```python
from build123d import *

# Parameters (mm, degrees)
SKETCH1_W                 = 15
SKETCH1_H                 = 15
BOSS_EXTRUDE1_DEPTH       = 3
SKETCH2_W                 = 8
SKETCH2_H                 = 3
CUT_EXTRUDE1_DEPTH        = 18.036725037
BOSS_EXTRUDE2_DEPTH       = 6
FILLET1_R                 = 2
CUT_EXTRUDE2_DEPTH        = 22.111371343
M3X0_5_TAPPED_HOLE1_D     = 2.5
M3X0_5_TAPPED_HOLE1_DEPTH = 7.5
M3X0_5_TAPPED_HOLE1_TIP   = 0.751075774
M3X0_5_TAPPED_HOLE2_D     = 2.5
M3X0_5_TAPPED_HOLE2_DEPTH = 7.5
M3X0_5_TAPPED_HOLE2_TIP   = 0.751075774


with BuildPart() as part:
    # Sketch1 → Boss-Extrude1 (new, symmetric)
    with BuildSketch(Plane.XY):
        Rectangle(SKETCH1_W, SKETCH1_H)
    extrude(amount=BOSS_EXTRUDE1_DEPTH, both=True)

    # Sketch2 → Cut-Extrude1 (cut, through all)
    with BuildSketch(Plane.XZ.offset(7.5)):
        Rectangle(SKETCH2_W, SKETCH2_H)
    extrude(amount=-CUT_EXTRUDE1_DEPTH, mode=Mode.SUBTRACT)

    # Sketch3 → Boss-Extrude2 (add)
    with BuildSketch(Plane.XY.offset(3)):
        with BuildLine():
            Line((7.5, -5.822370651), (7.5, 5.822370651))
            ThreePointArc((7.5, 5.822370651), (18.8, 0), (7.5, -5.822370651))
        make_face()
    extrude(amount=-BOSS_EXTRUDE2_DEPTH)

    # Fillet1
    # the kernel refuses this fillet: 2 mm, written as the material it adds along each edge
    with BuildSketch(Plane(origin=(7.5, -5.822370651, 3), x_dir=(0, -1, 0), z_dir=(0, 0, -1))) as fillet1_piece_1:
        with BuildLine():
            CenterArc((2.948715205, -1.544131065), FILLET1_R, 129.460264065, 67.086296359)
            ThreePointArc((1.031537969, -2.113719903), (0.603278499, -1.014153543), (0, 0))
            Line((0, 0), (1.677629349, 0))
        make_face()
    extrude(amount=6)
    with BuildSketch(Plane(origin=(7.5, 5.822370651, 3), x_dir=(0, 1, 0), z_dir=(0, 0, -1))) as fillet1_piece_2:
        with BuildLine():
            CenterArc((2.948715205, 1.544131065), FILLET1_R, 163.453439576, 67.086296359)
            ThreePointArc((1.031537969, 2.113719903), (0.603278499, 1.014153543), (0, 0))
            Line((0, 0), (1.677629349, 0))
        make_face()
    extrude(amount=6)
    # the kernel refuses this fillet: 2 mm, written as the material it takes off along each edge
    with BuildSketch(Plane(origin=(-7.5, -7.5, 8), x_dir=(1, 0, 0), z_dir=(0, 0, -1)), Plane(origin=(-7.5, 7.5, 8), x_dir=(0, -1, 0), z_dir=(0, 0, -1))) as fillet1_2_piece_1:
        with BuildLine():
            CenterArc((FILLET1_R, -FILLET1_R), FILLET1_R, 90, 90)
            Line((0, -FILLET1_R), (0, 0))
            Line((0, 0), (FILLET1_R, 0))
        make_face()
    extrude(amount=16, mode=Mode.SUBTRACT)

    # Sketch4 → Cut-Extrude2 (cut, through all)
    with BuildSketch(Plane(origin=(0, 0, -3), x_dir=(-1, 0, 0), z_dir=(0, 0, -1))):
        with BuildLine():
            Line((-18.8, 3), (-14.517490192, 3))
            ThreePointArc((-14.517490192, 3), (-7.5, 0), (-14.517490192, -3))
            Line((-14.517490192, -3), (-18.8, -3))
            Line((-18.8, -3), (-18.8, 3))
        make_face()
    extrude(amount=-CUT_EXTRUDE2_DEPTH, mode=Mode.SUBTRACT)

    # M3x0.5 Tapped Hole1
    with Locations(Plane(origin=(0, -7.5, 0), x_dir=(-1, 0, 0), z_dir=(0, -1, 0))):
        with Locations((-11.65, 0)):
            Hole(M3X0_5_TAPPED_HOLE1_D / 2, depth=M3X0_5_TAPPED_HOLE1_DEPTH)
            with Locations((0, 0, -(M3X0_5_TAPPED_HOLE1_DEPTH + M3X0_5_TAPPED_HOLE1_TIP / 2))):  # 118° drill point
                Cone(0, M3X0_5_TAPPED_HOLE1_D / 2, M3X0_5_TAPPED_HOLE1_TIP, mode=Mode.SUBTRACT)

    # M3x0.5 Tapped Hole2
    with Locations(Plane.XY.offset(3)):
        with Locations((0, 0)):
            Hole(M3X0_5_TAPPED_HOLE2_D / 2, depth=M3X0_5_TAPPED_HOLE2_DEPTH)
            with Locations((0, 0, -(M3X0_5_TAPPED_HOLE2_DEPTH + M3X0_5_TAPPED_HOLE2_TIP / 2))):  # 118° drill point
                Cone(0, M3X0_5_TAPPED_HOLE2_D / 2, M3X0_5_TAPPED_HOLE2_TIP, mode=Mode.SUBTRACT)


solid = part.part
```
For this review, take the finished solid that the model builds, in its own axes (mm). A direction names the side the tool comes from. Round coordinates to 2 decimals unless told otherwise and drop trailing zeros. Write each loop counter-clockwise with the first axis right and the second up, starting at its lowest first coordinate (ties: lowest second). Pieces come first, ordered by that corner, then holes. Notation, with made-up numbers: M 56.5,12.5 L 102.5,12.5 A18 cw 102.5,25.5 Z; hole C 59.25,61 d6. An arc over 180 degrees is marked long. One line per item, written item: value. Start each with the question number.
(1) We need section B-B (x = 11.65). Give the boundary of the cut face in (y, z), and give its area (3 significant figures).
(2) The part is to be moulded in two halves that separate along Y. For faces 1 (the cylindrical face through (7.5, 0.1, 0)), 2 (the flat face through (1, -7.5, 2)), 3 (the cylindrical face through (-6.93, 6.9, 0.04)), say which applies: released by +Y, released by -Y, zero draft, split by the parting line, or undercut.
(3) Insertion check: pin 1 (3 mm diameter, centred on x = 16, z = -0.5, fed in from +Y); pin 2 (2 mm diameter, centred on x = 11.65, z = 0, fed in from +Y); pin 3 (3 mm diameter, centred on x = 15.5, z = 1.5, fed in from -Y). Each pin has a flat end and moves straight along its axis. Give the tip position at first contact, or say it passes through.
(4) We need section D-D (y = 1.75). Give the boundary of the cut face in (x, z).
(5) Machinability: for faces 4 (the flat face through (16, -3, 0)), 5 (the cylindrical face through (14.53, 6.544, 0.042)), 6 (the flat face through (0, -2, 1.5)), 7 (the cylindrical face through (11.49, -5.53, -1.24)), which of the approach directions +Z, -Z, +X, -X, +Y, -Y give a long, thin tool a straight path to every point of the face, cutting with its end or side? Answer none if there is none.
(6) Wall thickness on line 1 (Z direction, x = -3.5, y = 6.5); line 2 (Y direction, x = 11.65, z = 1.75); line 3 (Z direction, x = 11.65, y = -4.9): over which ranges is each line inside the solid? List them lowest first.
(7) We need section A-A (x = -2). Give the boundary of the cut face in (y, z), and give its area (3 significant figures).
(8) We need section C-C (z = 1). Give the boundary of the cut face in (x, y).
Result:
1. outline: M -7.15,-3 L -4.15,-3 L -4.15,-1.25 L -7.15,-1.25 Z; M -7.15,1.25 L -4.15,1.25 L -4.15,3 L -7.15,3 Z; M 4.15,-3 L 7.15,-3 L 7.15,3 L 4.15,3 Z
1. area: 28.5 mm²
2. face 1: undercut
2. face 2: released by -Y
2. face 3: released by +Y
3. pin 1: y = 6.56
3. pin 2: y = 7.15
3. pin 3: y = -6.75
4. outline: M -7.5,-3 L 7.89,-3 L 7.89,3 L -7.5,3 Z; hole M -4,-1.5 L 4,-1.5 L 4,1.5 L -4,1.5 Z
5. face 4: +Z, -Z, +X
5. face 5: +Z, -Z, +Y
5. face 6: +Y, -Y
5. face 7: -Y
6. line 1: -3 to -1.5, 1.5 to 3
6. line 2: -7.15 to -4.15, 4.15 to 7.15
6. line 3: -3 to -1.25, 1.25 to 3
7. outline: M -7.5,-3 L 7.5,-3 L 7.5,-1.5 L -7.5,-1.5 Z; M -7.5,1.5 L 7.5,1.5 L 7.5,3 L -7.5,3 Z
7. area: 45.0 mm²
8. outline: M -7.5,-5.5 A2 ccw -5.5,-7.5 L -4,-7.5 L -4,7.5 L -5.5,7.5 A2 ccw -7.5,5.5 Z; M 4,-7.5 L 7.5,-7.5 A2 cw 9.61,-6.85 A7.15 ccw 10.9,-7.11 L 10.9,-4.08 A4.15 cw long 14.52,3 L 18.14,3 A7.15 ccw 9.61,6.85 A2 cw 7.5,7.5 L 4,7.5 Z; M 12.4,-7.11 A7.15 ccw 18.14,-3 L 14.52,-3 A4.15 cw 12.4,-4.08 Z
